```python
from build123d import *

# Parameters (mm, degrees)
BOSS_EXTRUDE1_DEPTH = 1.1
BOSS_EXTRUDE2_DEPTH = 17.8
BOSS_EXTRUDE3_DEPTH = 1.1
BOSS_EXTRUDE4_DEPTH = 20
LPATTERN1_COUNT     = 5
LPATTERN1_PITCH     = 5.86
BOSS_EXTRUDE5_DEPTH = 20
SKETCH7_W           = 6
SKETCH7_H           = 20
BOSS_EXTRUDE6_DEPTH = 7
SKETCH8_R           = 2.075
CUT_EXTRUDE1_DEPTH  = 14.1
SKETCH9_W           = 7.282395113
SKETCH9_H           = 2.9
BOSS_EXTRUDE7_DEPTH = 1.4


with BuildPart() as part:
    # Sketch2 → Boss-Extrude1 (new body)
    with BuildSketch(Plane(origin=(0, 0, 0), x_dir=(1, 0, 0), z_dir=(0, 1, 0))):
        Polygon((36, 15), (36, 4.881546635), (34.5, 4.881546635), (34.5, 15), (31, 15), (31, 4.881546635), (29.5, 4.881546635), (29.5, 15), (26, 15), (26, 4.881546635), (24.5, 4.881546635), (24.5, 15), (21, 15), (21, 4.881546635), (19.5, 4.881546635), (19.5, 15), (16, 15), (16, 4.881546635), (14.5, 4.881546635), (14.5, 15), (11, 15), (11, 4.881546635), (9.5, 4.881546635), (9.5, 15), (6, 15), (6, 6), (4.5, 6), (0, 6), (0, 0), (39.5, 0), (39.5, 15), align=None)
    extrude(amount=BOSS_EXTRUDE1_DEPTH)

    # Sketch3 → Boss-Extrude2 (add)
    with BuildSketch(Plane(origin=(0, 1.1, 0), x_dir=(1, 0, 0), z_dir=(0, 1, 0))):
        Polygon((6, 6), (0, 6), (0, 0), (39.5, 0), (39.5, 15), (36, 15), (36, 4.881546635), (34.5, 4.881546635), (34.5, 15), (31, 15), (31, 4.881546635), (29.5, 4.881546635), (29.5, 15), (26, 15), (26, 4.881546635), (24.5, 4.881546635), (24.5, 15), (21, 15), (21, 4.881546635), (19.5, 4.881546635), (19.5, 15), (16, 15), (16, 4.881546635), (14.5, 4.881546635), (14.5, 15), (11, 15), (11, 4.881546635), (9.5, 4.881546635), (9.5, 15), (6, 15), align=None)
        Polygon((7.1, 4.9), (7.1, 1.1), (38.4, 1.1), (38.4, 13.9), (37.1, 13.9), (37.1, 3.781546635), (33.4, 3.781546635), (33.4, 13.9), (32.1, 13.9), (32.1, 3.781546635), (28.4, 3.781546635), (28.4, 13.9), (27.1, 13.9), (27.1, 3.781546635), (23.4, 3.781546635), (23.4, 13.9), (22.1, 13.9), (22.1, 3.781546635), (18.4, 3.781546635), (18.4, 13.9), (17.1, 13.9), (17.1, 3.781546635), (13.4, 3.781546635), (13.4, 13.9), (12.1, 13.9), (12.1, 3.781546635), (8.4, 3.781546635), (8.4, 13.9), (7.1, 13.9), align=None, mode=Mode.SUBTRACT)
    extrude(amount=BOSS_EXTRUDE2_DEPTH)

    # Sketch4 → Boss-Extrude3 (add)
    with BuildSketch(Plane(origin=(0, 18.9, 0), x_dir=(1, 0, 0), z_dir=(0, 1, 0))):
        Polygon((0, 6), (0, 0), (39.5, 0), (39.5, 15), (36, 15), (36, 4.881546635), (34.5, 4.881546635), (34.5, 15), (31, 15), (31, 4.881546635), (29.5, 4.881546635), (29.5, 15), (26, 15), (26, 4.881546635), (24.5, 4.881546635), (24.5, 15), (21, 15), (21, 4.881546635), (19.5, 4.881546635), (19.5, 15), (16, 15), (16, 4.881546635), (14.5, 4.881546635), (14.5, 15), (11, 15), (11, 4.881546635), (9.5, 4.881546635), (9.5, 15), (6, 15), (6, 6), align=None)
    extrude(amount=BOSS_EXTRUDE3_DEPTH)

    # Sketch5 → Boss-Extrude4 (add)
    with BuildSketch(Plane.XZ):
        Polygon((33.440143193, 0), (39.5, 0), (38.775126266, 1.75), (39.5, 3.5), (33.440143193, 3.5), (32.715269459, 1.75), align=None)
        Polygon((33.014590612, 1.55), (35.897512895, 1.55), (35.381626855, 0.4), (34.816385288, 0.4), (33.490936209, 0.4), align=None, mode=Mode.SUBTRACT)
        Polygon((34.74142697, 3.1), (35.473359212, 3.1), (35.911102874, 1.95), (33.014590612, 1.95), (33.490936209, 3.1), align=None, mode=Mode.SUBTRACT)
        Polygon((35.820031028, 0.4), (36.420007202, 1.737451581), (35.901357695, 3.1), (38.901357695, 3.1), (38.342169386, 1.75), (38.901357695, 0.4), align=None, mode=Mode.SUBTRACT)
    boss_extrude4 = extrude(amount=-BOSS_EXTRUDE4_DEPTH)

    # LPattern1: Boss-Extrude4 ×5
    with Locations(*[(-i * LPATTERN1_PITCH, 0, 0) for i in range(1, LPATTERN1_COUNT)]):
        add(boss_extrude4)

    # Sketch6 → Boss-Extrude5 (add)
    with BuildSketch(Plane.XZ):
        Polygon((10.000143193, 3.5), (9.800143193, 3.5), (9.075269459, 1.75), (9.800143193, 0), (10.000143193, 0), (9.275269459, 1.75), align=None)
    extrude(amount=-BOSS_EXTRUDE5_DEPTH)

    # Sketch7 → Boss-Extrude6 (add)
    with BuildSketch(Plane.ZY):
        with Locations((-3, 10)):
            Rectangle(SKETCH7_W, SKETCH7_H)
    extrude(amount=BOSS_EXTRUDE6_DEPTH)

    # Sketch8 → Cut-Extrude1 (cut)
    with BuildSketch(Plane.ZY.offset(7)):
        with Locations((-3, 10)):
            Circle(SKETCH8_R)
    extrude(amount=-CUT_EXTRUDE1_DEPTH, mode=Mode.SUBTRACT)

    # Sketch9 → Boss-Extrude7 (add)
    with BuildSketch(Plane(origin=(0, 0, -6), x_dir=(-1, 0, 0), z_dir=(0, 0, -1))):
        with Locations((-2.358802444, 3.5)):
            Rectangle(SKETCH9_W, SKETCH9_H)
        with Locations((-2.358802444, 16.5)):
            Rectangle(SKETCH9_W, SKETCH9_H)
    extrude(amount=BOSS_EXTRUDE7_DEPTH)


solid = part.part
```
Geometry check sheet. Reference: the model listing, model coordinates, mm. A direction names the side the tool comes from. Give positions to 0.01 mm unless a question says otherwise; leave off trailing zeros. Order: outer loops, then holes, each group sorted by start corner. A loop starts at its lowest first (then second) coordinate and runs counter-clockwise, first axis right, second up.
1. Section check B-B, the plane z = -10.25. Give the number of separate pieces and of enclosed holes in the cut face, and give its area (3 significant figures).
2. Access from +Z, -Z, +X, -X, +Y, -Y to the whole of each face (thin tool, end or side, straight path). Record for faces 1 (the face through (2, 4.95, -7)), 2 (the face through (20, 10, -4.882)), 3 (the face through (17, 10, 3.1)), 4 (the face through (39.13, 9.86, 2.61)).
3. Release check for a two-part mould opening along Y. For faces 5 (the face through (37, 10, 3.1)), 6 (the face through (22.1, 10, -9)) record: pulls with the +Y half, pulls with the -Y half, needs draft (parallel to the pull), parting line crosses it, or undercut.
4. Section check A-A, the plane x = 3. Enter the section's corners in (y, z) (3 decimals), and give its area (3 significant figures).
5. Thickness scan on L1, parallel to Z at x = 37.5, y = 11.75; L2, parallel to Z at x = 13.5, y = 7.5; L3, parallel to Z at x = 11.5, y = 13.75. Record the ranges inside material, lowest first.
6. Gauge pin test, flat ends, axial feed: pin 1 Ø0.9 at (x, y) = (25, 14) entering from -Z; pin 2 Ø3 at (x, y) = (3.5, 3.5) entering from -Z; pin 3 Ø4 at (x, y) = (1, 12) entering from -Z. Record the tip position at first contact, or that the pin passes through.
7. Section check C-C, the plane z = -3. Enter the section's corners in (x, y) (3 decimals).
Values follow:
1. separate pieces: 7
1. enclosed holes: 7
1. area: 328 mm2
2. face 1: -Z, -X
2. face 2: -Z, +Y, -Y
2. face 3: +Y, -Y
2. face 4: +X, +Y, -Y
3. face 5: needs draft
3. face 6: undercut
4. outline: (0, -6) - (2.05, -6) - (2.05, -7.4) - (4.95, -7.4) - (4.95, -6) - (15.05, -6) - (15.05, -7.4) - (17.95, -7.4) - (17.95, -6) - (20, -6) - (20, 0) - (0, 0) - close; hole circle Ø4.15 at (10, -3)
4. area: 115 mm2
5. L1: z = -15 to -13.9, -1.1 to 0.4, 3.1 to 3.5
5. L2: z = -15 to -3.78, -1.1 to 0.4, 3.1 to 3.5
5. L3: z = -15 to -3.78, -1.1 to 0.4, 1.55 to 1.95, 3.1 to 3.5
6. pin 1: stops at z = -4.88
6. pin 2: stops at z = -7.4
6. pin 3: stops at z = -6
7. outline: (-7, 0) - (39.5, 0) - (39.5, 20) - (-7, 20) - (-7, 12.075) - (7.1, 12.075) - (7.1, 18.9) - (38.4, 18.9) - (38.4, 1.1) - (7.1, 1.1) - (7.1, 7.925) - (-7, 7.925) - close
